Input: part model. Units: mm. Frame: model coordinates. Face numbers are marked on the shaded views. A direction names the side the tool comes from. Coordinates: 2 decimals unless noted, no trailing zeros. Loops run counter-clockwise (first coordinate to the right, second up) from the corner with the lowest first, then second, coordinate; pieces in that order, holes last. Notation, with made-up numbers: (36, -5.5) - (46, -5.5) arc R11 ccw to (46, 7.5) - close; hole circle Ø7 at (-34, 29). An arc over 180 degrees is marked (long way). Use a Markdown table: item, result. Add a question column.
1. Ray query, L1, parallel to Z at x = -12, y = -55.5; L2, parallel to Z at x = -21, y = -13; L3, parallel to X at y = -71.5, z = 12.5. Return the intervals inside material, ascending. Write a range as [from, to].
2. Section query A-A on z = -20.5. Return the cut outline in (x, y), then the cut area to 3 significant figures.
3. Section query B-B on x = 6. Return the cut outline in (y, z).
4. Section query C-C on y = -93. Return the cut outline in (x, z), then the cut area to 3 significant figures.
5. Contact query for flat-ended pins moving along their axis: P1, Ø0.5, axis at y = -25.5, z = 25, coming from the +X side; P2, Ø1, axis at y = -79, z = 19.5, coming from the +X side; P3, Ø1.5, axis at y = -41, z = 18, coming from the +X side; P4, Ø12, axis at x = 17.5, y = -120, coming from the +Z side. Output: stop coordinate, or through.
6. Access query for the marked faces 4 and 5. Directions: +Z, -Z, +X, -X, +Y, -Y. A direction counts if a zero-diameter tool reaches every point of the face in a straight line with its end or side. Return the directions, or none.
7. Section query D-D on y = -33. Return the cut outline in (x, z), then the cut area to 3 significant figures.
8. Draft query along Z for the marked faces 1, 2 and 3. Return one class per face: released by +Z, released by -Z, zero draft, split by the parting line, or undercut.
```python
from build123d import *

# Parameters (mm, degrees)
F1_DEPTH = 160
F2_DEPTH = 140
F4_DEPTH = 1.4817621135
F6_DEPTH = 5


# Not quite as in the source:
# - a feature names something its author has since deleted; it is built from what else it names


with BuildPart() as f1:
    # F0 (on Front) → F1 (new body)
    with BuildSketch(Plane.XZ):
        Polygon((14.7224318643, 25.5), (-14.7224318643, 25.5), (-29.4448637287, 0), (-14.7224318643, -25.5), (14.7224318643, -25.5), (29.4448637287, 0), align=None)
        Polygon((-28.8675134595, 0), (-14.4337567297, 25), (14.4337567297, 25), (28.8675134595, 0), (14.4337567297, -25), (12.7224318643, -25), (-12.7224318643, -25), (-14.4337567297, -25), align=None, mode=Mode.SUBTRACT)
    extrude(amount=F1_DEPTH)

    # F0 (on Front) → F2 (join)
    with BuildSketch(Plane.XZ):
        Polygon((14.7224318643, 25.5), (-14.7224318643, 25.5), (-29.4448637287, 0), (-14.7224318643, -25.5), (14.7224318643, -25.5), (29.4448637287, 0), align=None)
        Polygon((-28.8675134595, 0), (-14.4337567297, 25), (14.4337567297, 25), (28.8675134595, 0), (14.4337567297, -25), (12.7224318643, -25), (-12.7224318643, -25), (-14.4337567297, -25), align=None, mode=Mode.SUBTRACT)
    extrude(amount=F2_DEPTH)

    # F3 (on face) → F4 (cut, through all)
    with BuildSketch(Plane(origin=(22.0836477965, 0, 12.75), x_dir=(0, 1, 0), z_dir=(0.8660254038, 0, 0.5))):
        with BuildLine():
            ThreePointArc((-130.0384322302, -14.7224318643), (-121.3330579218, -9.537184599), (-117.9107135534, 0))
            ThreePointArc((-117.9107135534, 0), (-121.3330579218, 9.537184599), (-130.0384322302, 14.7224318643))
            Line((-130.0384322302, 14.7224318643), (-135.7829948767, 14.7224318643))
            ThreePointArc((-135.7829948767, 14.7224318643), (-147.9107135534, 0), (-135.7829948767, -14.7224318643))
            Line((-135.7829948767, -14.7224318643), (-130.0384322302, -14.7224318643))
        make_face()
        with BuildLine():
            ThreePointArc((-135.7829948767, -14.7224318643), (-132.9107135534, -15), (-130.0384322302, -14.7224318643))
            Line((-130.0384322302, -14.7224318643), (-135.7829948767, -14.7224318643))
        make_face()
        with BuildLine():
            Line((-135.7829948767, 14.7224318643), (-130.0384322302, 14.7224318643))
            ThreePointArc((-130.0384322302, 14.7224318643), (-132.9107135534, 15), (-135.7829948767, 14.7224318643))
        make_face()
    extrude(amount=-F4_DEPTH, mode=Mode.SUBTRACT)

    # F5 (on face) → F6 (cut)
    with BuildSketch(Plane.XY.offset(25.5)):
        with BuildLine():
            Line((14.7224318643, -28.900016646), (14.7224318643, -23.1554539994))
            ThreePointArc((14.7224318643, -23.1554539994), (0, -11.0277353227), (-14.7224318643, -23.1554539994))
            Line((-14.7224318643, -23.1554539994), (-14.7224318643, -28.900016646))
            ThreePointArc((-14.7224318643, -28.900016646), (0, -41.0277353227), (14.7224318643, -28.900016646))
        make_face()
    extrude(amount=-F6_DEPTH, mode=Mode.SUBTRACT)


solid = f1.part
```
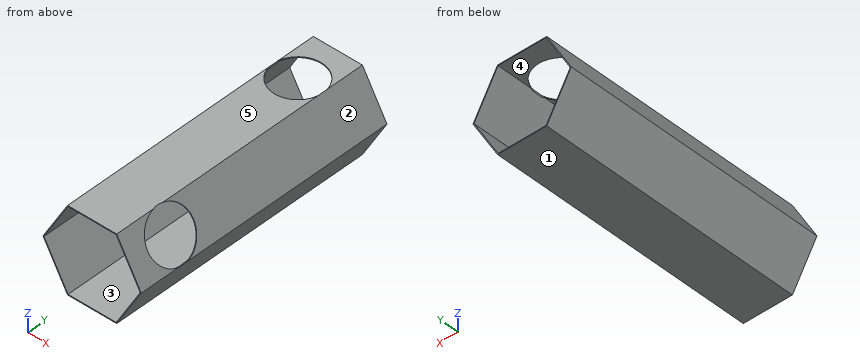
Resolved:
| question | item | result |
|---|---|---|
| 1 | L1 | [-25.5, -25], [25, 25.5] |
| 1 | L2 | [-14.63, -13.63], [13.63, 14.63] |
| 1 | L3 | [-22.23, -21.65], [21.65, 22.23] |
| 2 | outline | (-17.61, -160) - (-17.03, -160) - (-17.03, 0) - (-17.61, 0) - close; (17.03, -160) - (17.61, -160) - (17.61, 0) - (17.03, 0) - close |
| 2 | area | 185 mm² |
| 3 | outline | (-160, -25.5) - (0, -25.5) - (0, -25) - (-160, -25) - close; (-160, 25) - (-39.78, 25) - (-39.78, 25.5) - (-160, 25.5) - close; (-12.28, 25) - (0, 25) - (0, 25.5) - (-12.28, 25.5) - close |
| 4 | outline | (-29.44, 0) - (-14.72, -25.5) - (14.72, -25.5) - (29.44, 0) - (14.72, 25.5) - (-14.72, 25.5) - close; hole (-28.87, 0) - (-14.43, -25) - (14.43, -25) - (28.87, 0) - (14.43, 25) - (-14.43, 25) - close |
| 4 | area | 87.5 mm² |
| 5 | P1 | x = 15.16 |
| 5 | P2 | x = 18.48 |
| 5 | P3 | x = 19.49 |
| 5 | P4 | z = 25.5 |
| 6 | face 4 | +Y, -Y |
| 6 | face 5 | +Z, +X, -X, +Y, -Y |
| 7 | outline | (-29.44, 0) - (-14.72, -25.5) - (14.72, -25.5) - (29.44, 0) - (14.72, 25.5) - (13.28, 25.5) - (13.28, 25) - (14.43, 25) - (28.87, 0) - (14.43, -25) - (-14.43, -25) - (-28.87, 0) - (-14.43, 25) - (-13.28, 25) - (-13.28, 25.5) - (-14.72, 25.5) - close |
| 7 | area | 74.2 mm² |
| 8 | face 1 | released by -Z |
| 8 | face 2 | released by +Z |
| 8 | face 3 | undercut |
